Part model, mm, in its own coordinate system. A direction names the side the tool comes from. Coordinates: 2 decimals unless noted, no trailing zeros. Write each loop counter-clockwise with the first axis right and the second up, starting at its lowest first coordinate (ties: lowest second). Pieces come first, ordered by that corner, then holes. Notation, with made-up numbers: (65, -10.75) - (88, -10.75) arc R18 ccw to (88, 4.25) - close; hole circle Ø6 at (-5, 7). An arc over 180 degrees is marked (long way). Use one line per item in the form item = value. Start each with the question number.
Autodesk Inventor part; units mm, degrees
ref_plane "YZ Plane" through (0, 0, 0) normal (1, 0, 0) x (0, 1, 0)
ref_plane "XZ Plane" through (0, 0, 0) normal (0, 1, 0) x (-1, 0, 0)
ref_plane "XY Plane" through (0, 0, 0) normal (0, 0, 1) x (1, 0, 0)
sketch "Szkic1" plane through (0, 0, 0) normal (1, 0, 0) x (0, 1, 0)
  line L0 (0, 0) -> (-49.134, 0)
  line L1 (-49.134, 1) -> (0, 1)
  line L2 (0, 1) -> (0, 0)
  circle A0 centre (-50, 0.5) radius 1
  circle A1 centre (-50, 0.5) radius 0.5
  dimension "d0" = 2
  dimension "d1" = 1
  dimension "d2" = 49.134
  dimension "d3" = 1
extrude "Wyciągnięcie proste1" add sketch "Szkic1" along normal blind 50 contours L0 A0 L1 L2
extrude "Wyciągnięcie proste2" add sketch "Szkic1" along normal blind 50 contours A1
extrude "Wyciągnięcie proste3" add sketch "Szkic1" along normal blind 25 contours A0
properties part number "zawias2"
Q1. Slice it at A-A (x = 32). List the corners of the cut face in (y, z), plus the area to 3 significant figures.
Q2. Slice it at B-B (y = -22). List the corners of the cut face in (x, z).
Q3. Which spindle directions (+Z, -Z, +X, -X, +Y, -Y) get a long thin tool onto all of the face, cutting with end or side? Do faces 1 (the flat face through (25, -24, 0)), 2 (the cylindrical face through (12.3, -51, 0.5)), 3 (the flat face through (25, -25, 1)). Say none if no direction does.
Q4. Slice it at C-C (x = 20). List the corners of the cut face in (y, z).
Q5. Drill centre lines: probe 1 along Z at (x, y) = (12, -31); probe 2 along Y at (x, z) = (5, 0.55); probe 3 along Y at (x, z) = (38, 0.85). Where is each one in solid material? Low to high.
Q6. Pin check, flat tips, straight feed: P1, Ø5, axis at x = 21.5, y = -29.5, coming from the +Z side; P2, Ø14.5, axis at x = 28.5, y = -19.5, coming from the -Z side. Stop position of each tip, or through.
Solution:
q1.outline = circle Ø1 at (-50, 0.5); (-49.13, 0) - (0, 0) - (0, 1) - (-49.13, 1) arc R1 cw to start
q1.area = 49.8 mm2
q2.outline = (0, 0) - (50, 0) - (50, 1) - (0, 1) - close
q3.face_1 = -Z, +X, -X, +Y
q3.face_2 = +X, -X
q3.face_3 = +Z, +X, -X, +Y
q4.outline = (-49.13, 0) - (0, 0) - (0, 1) - (-49.13, 1) arc R1 ccw (long way) to start
q5.probe_1 = 0 to 1
q5.probe_2 = -51 to 0
q5.probe_3 = -50.36 to -49.64, -49.06 to 0
q6.P1 = 1
q6.P2 = 0
